```python
from build123d import *

# Parameters (mm, degrees)
SKETCH2_R           = 14
SKETCH2_R_2         = 8
BOSS_EXTRUDE2_DEPTH = 7.5
SKETCH5_R           = 1.15
CUT_EXTRUDE2_DEPTH  = 22.17191536
SKETCH7_R           = 1.75
CUT_EXTRUDE3_DEPTH  = 7
SKETCH9_R           = 1.75
CUT_EXTRUDE4_DEPTH  = 7


with BuildPart() as part:
    # Sketch2 → Boss-Extrude2 (new body)
    with BuildSketch(Plane.XY.offset(2)):
        Circle(SKETCH2_R)
        Circle(SKETCH2_R_2, mode=Mode.SUBTRACT)
    extrude(amount=BOSS_EXTRUDE2_DEPTH)

    # Sketch5 → Cut-Extrude2 (cut, through all)
    with BuildSketch(Plane.XY.offset(9.5)):
        with Locations((0, 10.85)):
            Circle(SKETCH5_R)
        with Locations((10.85, 0)):
            Circle(SKETCH5_R)
        with Locations((0, -10.85)):
            Circle(SKETCH5_R)
        with Locations((-10.85, 0)):
            Circle(SKETCH5_R)
    extrude(amount=-CUT_EXTRUDE2_DEPTH, mode=Mode.SUBTRACT)

    # Sketch7 → Cut-Extrude3 (cut)
    with BuildSketch(Plane(origin=(9.899494937, 9.899494937, 0), x_dir=(0.7071067811865489, -0.7071067811865461, 0), z_dir=(0.7071067811865461, 0.7071067811865489, 0))):
        with Locations(Location((0, -5.75, 0), (0, 0, 180))):
            Circle(SKETCH7_R)
    extrude(amount=-CUT_EXTRUDE3_DEPTH, mode=Mode.SUBTRACT)

    # Sketch9 → Cut-Extrude4 (cut)
    with BuildSketch(Plane(origin=(-9.899494937, 9.899494937, 0), x_dir=(0, 0, 1), z_dir=(-0.7071067811865489, 0.7071067811865462, 0))):
        with Locations(Location((5.75, 0, 0), (0, 0, 270))):
            Circle(SKETCH9_R)
    extrude(amount=-CUT_EXTRUDE4_DEPTH, mode=Mode.SUBTRACT)


solid = part.part
```
Check sheet for the modelled part. Datum: model origin and axes. Units: mm. Coordinates: 2 decimals unless noted, no trailing zeros. Order: outer loops, then holes, each group sorted by start corner. A loop starts at its lowest first (then second) coordinate and runs counter-clockwise, first axis right, second up. Notation, with made-up numbers: M -19,42 L 31,42 A16 cw 31,66 Z; hole C -5,41.25 d10. An arc over 180 degrees is marked long. Write each question's results on one line, items separated by ' | '. Start each with the question number.
1. Cross-section at D-D on y = -7. Record the cut outline in (x, z).
2. Cross-section at B-B on z = 4.75. Record the cut outline in (x, y).
3. Go/stop test with flat-tipped pins: P1, Ø1.5, axis at y = 7, z = 4.5, coming from the -X side; P2, Ø9.5, axis at x = 0, y = 0, coming from the -Z side; P3, Ø3, axis at x = 6, z = 4.5, coming from the +Y side; P4, Ø1, axis at y = -2.5, z = 8, coming from the +X side. Record where each tip stops, or that it passes through.
4. Cross-section at A-A on x = 0. Record the cut outline in (y, z), and give its area (3 significant figures).
5. Material ranges on probe 1 along Y at (x, z) = (0, 6.25); probe 2 along X at (y, z) = (7, 5.25); probe 3 along Y at (x, z) = (-10.5, 8.75), recorded low to high.
6. Mould release check, pull along Y, two halves, no side actions. Record for faces 1 (the face through (6.5, -12.4, 5.7)), 2 (the face through (6, -6, 2)), 3 (the face through (9.7, 0.05, 5.8)): +Y half, -Y half, draft (parallel to the pull), parting line (faces both ways), or undercut.
Checks:
1) outline: M -12.12,2 L -3.87,2 L -3.87,9.5 L -12.12,9.5 Z; M 3.87,2 L 12.12,2 L 12.12,9.5 L 3.87,9.5 Z
2) outline: M -10.86,8.83 A14 ccw long 10.86,8.83 L 6.58,4.55 A8 cw long -6.58,4.55 Z; M -8.83,10.86 L -4.55,6.58 A8 cw 4.55,6.58 L 8.83,10.86 A14 ccw Z; hole C -10.85,0 d2.3; hole C 0,-10.85 d2.3; hole C 0,10.85 d2.3; hole C 10.85,0 d2.3
3) P1: stops at x = -12.53 | P2: passes through | P3: stops at y = 13.26 | P4: stops at x = 13.86
4) outline: M -14,2 L -12,2 L -12,9.5 L -14,9.5 Z; M -9.7,2 L -8,2 L -8,9.5 L -9.7,9.5 Z; M 8,2 L 9.7,2 L 9.7,9.5 L 8,9.5 Z; M 12,2 L 14,2 L 14,9.5 L 12,9.5 Z | area: 55.5 mm²
5) probe 1: y = -14 to -12, -9.7 to -8, 8 to 9.7, 12 to 14 | probe 2: x = -12.12 to -9.37, -4.63 to -3.87, 3.87 to 4.63, 9.37 to 12.12 | probe 3: y = -9.26 to -1.1, 1.1 to 9.26
6) face 1: parting line | face 2: draft | face 3: undercut
